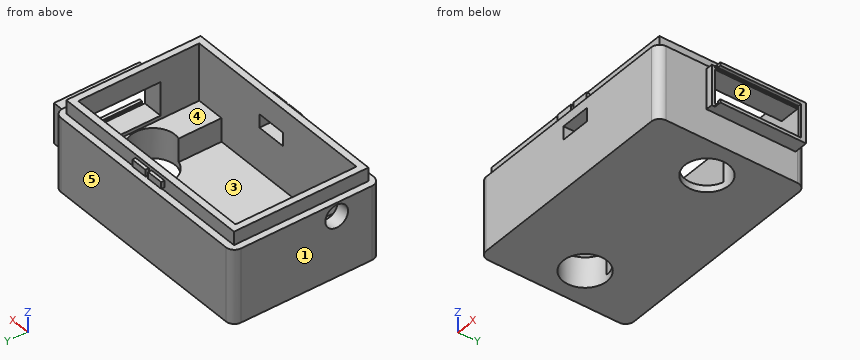
from build123d import *

# Parameters (mm, degrees)
SKETCH1_W                   = 68
SKETCH1_H                   = 44
MIAN_BOSS_EXTRUDE_DEPTH     = 26
SKETCH2_W                   = 60
SKETCH2_H                   = 36
MAIN_CUT_DEPTH              = 17
SKETCH4_W                   = 45
SKETCH4_H                   = 35
BATTERY_CUT_DEPTH           = 7
SKETCH5_R                   = 6.5
ELCTRODE_CUT_DEPTH          = 12
SKETCH6_W                   = 9.989337028
SKETCH6_H                   = 24.5
USB_C_CUT_DEPTH             = 7
SKETCH7_R                   = 3.375
BUTTON_CUT_DEPTH            = 7
SKETCH8_W                   = 9
SKETCH8_H                   = 4
SWITCH_CUT_DEPTH            = 7
OUTSIDE_FILLET_R            = 2.5
SKETCH10_OUTSIDE_W          = 87.012
SKETCH10_OUTSIDE_H          = 63.012
SKETCH10_OUTSIDE_W_2        = 64
SKETCH10_OUTSIDE_H_2        = 40
OUTER_LID_EXTRUDE_DEPTH     = 4
LID_SNAP_EXTRUDE_DEPTH      = 1
LID_SNAP_EXTRUDE_DEPTH_BACK = 41
SKETCH11_W                  = 5
SKETCH11_H                  = 2
SKETCH13_W                  = 11
SKETCH13_H                  = 36
INNER_LID_EXTRUDE_DEPTH     = 3
SKETCH14_W                  = 11.989337028
SKETCH14_H                  = 26.5
SKETCH14_W_2                = 9.989337028
SKETCH14_H_2                = 24.5
USB_COVER_EXTRUDE_DEPTH     = 4
SKETCH15_W                  = 11.989337028
SKETCH15_H                  = 1
USB_CUT_EXTRUDE_DEPTH       = 2
USB_LIP_CUT_DEPTH           = 10.5
USB_LIP_CUT_DEPTH_BACK      = 0.5
SKETCH18_W                  = 1
SKETCH18_H                  = 24.5
SKETCH20_W                  = 1
SKETCH20_H                  = 9.989337028
USB_LIP_BOSS_DEPTH          = 0.5


with BuildPart() as part:
    # Sketch1 → Mian Boss Extrude (new body)
    with BuildSketch(Plane.XY):
        with Locations((34, 22)):
            Rectangle(SKETCH1_W, SKETCH1_H)
    extrude(amount=MIAN_BOSS_EXTRUDE_DEPTH)

    # Sketch2 → Main cut (cut)
    with BuildSketch(Plane.XY.offset(26)):
        with Locations((34, 22)):
            Rectangle(SKETCH2_W, SKETCH2_H)
    extrude(amount=-MAIN_CUT_DEPTH, mode=Mode.SUBTRACT)

    # Sketch4 → Battery Cut (cut)
    with BuildSketch(Plane.XY.offset(9)):
        with Locations((33, 21.5)):
            Rectangle(SKETCH4_W, SKETCH4_H)
    extrude(amount=-BATTERY_CUT_DEPTH, mode=Mode.SUBTRACT)

    # Sketch5 → Elctrode Cut (cut)
    with BuildSketch(Plane(origin=(0, 0, 0), x_dir=(-1, 0, 0), z_dir=(0, 0, -1))):
        with Locations((-57.25, 23)):
            Circle(SKETCH5_R)
        with Locations((-10.75, 23)):
            Circle(SKETCH5_R)
    extrude(amount=-ELCTRODE_CUT_DEPTH, mode=Mode.SUBTRACT)

    # Sketch6 → USB-c Cut (cut)
    with BuildSketch(Plane(origin=(68, 0, 0), x_dir=(0, 0, -1), z_dir=(1, 0, 0))):
        with Locations((-15.005331486, 27.75)):
            Rectangle(SKETCH6_W, SKETCH6_H)
    extrude(amount=-USB_C_CUT_DEPTH, mode=Mode.SUBTRACT)

    # Sketch7 → Button Cut (cut)
    with BuildSketch(Plane.ZY):
        with Locations((18, 13)):
            Circle(SKETCH7_R)
    extrude(amount=-BUTTON_CUT_DEPTH, mode=Mode.SUBTRACT)

    # Sketch8 → Switch Cut (cut)
    with BuildSketch(Plane.XZ):
        with Locations((36.5, 17)):
            Rectangle(SKETCH8_W, SKETCH8_H)
    extrude(amount=-SWITCH_CUT_DEPTH, mode=Mode.SUBTRACT)

    # Outside Fillet
    outside_fillet_edges = [part.edges().sort_by_distance(p)[0] for p in [
        (0, 44, 13),
        (68, 44, 13),
        (68, 0, 13),
        (0, 0, 13),
    ]]
    fillet(outside_fillet_edges, radius=OUTSIDE_FILLET_R)

    # Sketch10 outside → Outer lid Extrude (cut)
    with BuildSketch(Plane.XY.offset(26)):
        with Locations((34, 22)):
            Rectangle(SKETCH10_OUTSIDE_W, SKETCH10_OUTSIDE_H)
        with Locations((34, 22)):
            Rectangle(SKETCH10_OUTSIDE_W_2, SKETCH10_OUTSIDE_H_2, mode=Mode.SUBTRACT)
    extrude(amount=-OUTER_LID_EXTRUDE_DEPTH, mode=Mode.SUBTRACT)

    # Sketch11 → Lid Snap-Extrude (add, two sides: drawn at the far end of the back side and taken through both)
    with BuildSketch(Plane.XZ.offset(-2).offset(-LID_SNAP_EXTRUDE_DEPTH_BACK)):
        with Locations((31, 24)):
            Rectangle(SKETCH11_W, SKETCH11_H)
        with Locations((37, 24)):
            Rectangle(SKETCH11_W, SKETCH11_H)
    extrude(amount=LID_SNAP_EXTRUDE_DEPTH + LID_SNAP_EXTRUDE_DEPTH_BACK)

    # Sketch13 → Inner Lid-Extrude (cut)
    with BuildSketch(Plane.XY.offset(25)):
        with Locations((34, 22)):
            Rectangle(SKETCH13_W, SKETCH13_H)
    extrude(amount=-INNER_LID_EXTRUDE_DEPTH, mode=Mode.SUBTRACT)

    # Sketch14 → USB Cover-Extrude (add)
    with BuildSketch(Plane(origin=(68, 0, 0), x_dir=(0, 0, -1), z_dir=(1, 0, 0))):
        with Locations((-15.005331486, 27.75)):
            Rectangle(SKETCH14_W, SKETCH14_H)
        with Locations((-15.005331486, 27.75)):
            Rectangle(SKETCH14_W_2, SKETCH14_H_2, mode=Mode.SUBTRACT)
    extrude(amount=USB_COVER_EXTRUDE_DEPTH)

    # Sketch15 → USB Cut-Extrude (cut)
    with BuildSketch(Plane(origin=(72, 0, 0), x_dir=(0, 0, -1), z_dir=(1, 0, 0))):
        with Locations((-15.005331486, 15)):
            Rectangle(SKETCH15_W, SKETCH15_H)
    extrude(amount=-USB_CUT_EXTRUDE_DEPTH, mode=Mode.SUBTRACT)

    # Sketch18 → USB Lip Cut (cut, two sides: drawn at the far end of the back side and taken through both)
    with BuildSketch(Plane(origin=(0, 0, 20), x_dir=(-1, 0, 0), z_dir=(0, 0, -1)).offset(-USB_LIP_CUT_DEPTH_BACK)):
        with Locations((-70.5, 27.75)):
            Rectangle(SKETCH18_W, SKETCH18_H)
    extrude(amount=USB_LIP_CUT_DEPTH + USB_LIP_CUT_DEPTH_BACK, mode=Mode.SUBTRACT)

    # Sketch20 → USB Lip Boss (add)
    with BuildSketch(Plane.XZ.offset(-40)):
        with Locations((71.5, 15.005331486)):
            Rectangle(SKETCH20_W, SKETCH20_H)
    extrude(amount=USB_LIP_BOSS_DEPTH)


solid = part.part
Design review of the part built by this model. Coordinates are the model's own, in mm. Face numbers are marked on the shaded views. A direction names the side the tool comes from. Give positions to 0.01 mm unless a question says otherwise; leave off trailing zeros. Order: outer loops, then holes, each group sorted by start corner. A loop starts at its lowest first (then second) coordinate and runs counter-clockwise, first axis right, second up. Notation, with made-up numbers: (-30.5, 25.5) - (-4.5, 25.5) arc R23 cw to (-4.5, 61.5) - close; hole circle Ø10 at (83.5, 2). An arc over 180 degrees is marked (long way). Write item = value, one per line. Start each with the question number.
Q1. We need section D-D on z = 24. State the section outline as (x, y) points.
Q2. To check wall thickness, follow L1, parallel to X at y = 26, z = 20.25; L2, parallel to X at y = 7, z = 11.5; L3, parallel to Y at x = 57.25, z = 6. State the ranges of each line that lie inside material, in increasing order. Write a range as from..to.
Q3. Clearance check with flat-ended pins moving along their axes: pin 1 Ø1.6 at (x, z) = (36, 24) entering from -Y; pin 2 Ø0.8 at (y, z) = (42.5, 24.5) entering from -X; pin 3 Ø0.5 at (x, y) = (31.5, 1.5) entering from +Z. State where each tip first meets the part, or that it passes through.
Q4. We need section A-A on z = 18. State the section outline as (x, y) points (3 decimals), plus the area to 3 significant figures.
Q5. Mouldability with a two-part tool opening along Z and no side actions: class the marked faces 1, 2 and 3 as released by +Z, released by -Z, zero draft, split by the parting line, or undercut.
Q6. We need section C-C on x = 67. State the section outline as (y, z) points.
Q7. Tool access review of the marked faces 4 and 5: name each direction out of +Z, -Z, +X, -X, +Y, -Y from which nothing blocks a thin tool from reaching the whole face with its end or side.
Working result:
q1.outline = (2, 2) - (28.5, 2) - (28.5, 1) - (33.5, 1) - (33.5, 2) - (34.5, 2) - (34.5, 1) - (39.5, 1) - (39.5, 2) - (66, 2) - (66, 42) - (39.5, 42) - (39.5, 43) - (34.5, 43) - (34.5, 42) - (33.5, 42) - (33.5, 43) - (28.5, 43) - (28.5, 42) - (2, 42) - close; hole (4, 4) - (64, 4) - (64, 40) - (4, 40) - close
q2.L1 = 0..4, 64..70, 71..72
q2.L2 = 0..4, 64..68
q2.L3 = 0..16.5, 29.5..44
q3.pin_1 = 1
q3.pin_2 = 28.5
q3.pin_3 = 25
q4.outline = (0, 2.5) arc R2.5 ccw to (2.5, 0) - (32, 0) - (32, 4) - (4, 4) - (4, 9.625) - (0, 9.625) - close; (0, 16.375) - (4, 16.375) - (4, 40) - (71, 40) - (71, 39.5) - (72, 39.5) - (72, 41) - (68, 41) - (68, 41.5) arc R2.5 ccw to (65.5, 44) - (2.5, 44) arc R2.5 ccw to (0, 41.5) - close; (41, 0) - (65.5, 0) arc R2.5 ccw to (68, 2.5) - (68, 14.5) - (70, 14.5) - (70, 15.5) - (64, 15.5) - (64, 4) - (41, 4) - close
q4.area = 672 mm²
q5.face_1 = zero draft
q5.face_2 = undercut
q5.face_3 = released by +Z
q6.outline = (0.5, 0) - (43.5, 0) - (43.5, 22) - (0.5, 22) - close; hole (15.5, 10.01) - (40, 10.01) - (40, 20) - (15.5, 20) - close
q7.face_4 = +Z
q7.face_5 = +Z, -Z, +X, -X, +Y
